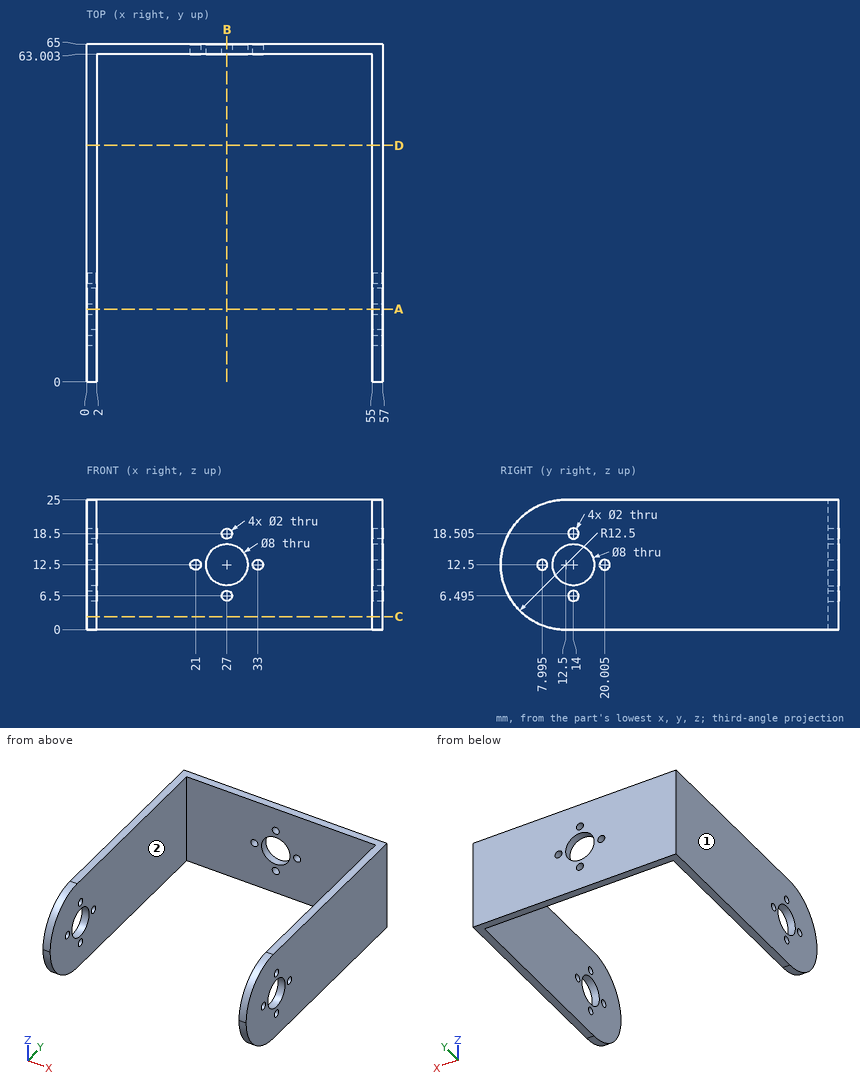
Could you check a few things on this drawing? It's one solid part, dimensions in mm from its lowest x, y, z. A direction names the side the tool comes from. Give positions to 0.01 mm unless a question says otherwise; leave off trailing zeros. Order: outer loops, then holes, each group sorted by start corner. A loop starts at its lowest first (then second) coordinate and runs counter-clockwise, first axis right, second up. Notation, with made-up numbers: (72, 37.25) -> (102, 37.25) arc R23 ccw to (102, 72.25) -> close; hole circle Ø5 at (50, -37). An arc over 180 degrees is marked (long way). Answer in a Markdown table with one row per item. Add a question column.
Item 1: Imagine slicing it at C-C (z = 2.5). List the corners of the cut face in (x, y) for me.
Item 2: I'm going to push a flat-ended pin straight in: P1, Ø3, axis at x = 27, z = 6.5, coming from the -Y side. Where does the tip first touch, or does it pass through?
Item 3: For the marked faces 1 and 2, which set-ups out of +Z, -Z, +X, -X, +Y, -Y let a thin tool reach every point of the face, with its end or its side?
Item 4: Imagine slicing it at B-B (x = 27). List the corners of the cut face in (y, z) for me.
Item 5: Please list where these lines run through material, in increasing order: probe 1 along X at (y, z) = (60.5, 12); probe 2 along Y at (x, z) = (49, 17.5).
Item 6: Imagine slicing it at D-D (y = 45.5). List the corners of the cut face in (x, z) for me, and give its area (3 significant figures).
Item 7: Imagine slicing it at A-A (y = 14). Count the separate pieces of the cut face and the enclosed holes in it.
Result:
| question | item | result |
|---|---|---|
| 1 | outline | (0, 5) -> (2, 5) -> (2, 63) -> (55, 63) -> (55, 5) -> (57, 5) -> (57, 65) -> (0, 65) -> close |
| 2 | P1 | y = 63 |
| 3 | face 1 | +Z, -Z, -X, +Y, -Y |
| 3 | face 2 | +Z, -Z, -Y |
| 4 | outline | (63, 0) -> (65, 0) -> (65, 5.5) -> (63, 5.5) -> close; (63, 7.5) -> (65, 7.5) -> (65, 8.5) -> (63, 8.5) -> close; (63, 16.5) -> (65, 16.5) -> (65, 17.5) -> (63, 17.5) -> close; (63, 19.5) -> (65, 19.5) -> (65, 25) -> (63, 25) -> close |
| 5 | probe 1 | 0 to 2, 55 to 57 |
| 5 | probe 2 | 63 to 65 |
| 6 | outline | (0, 0) -> (2, 0) -> (2, 25) -> (0, 25) -> close; (55, 0) -> (57, 0) -> (57, 25) -> (55, 25) -> close |
| 6 | area | 100 mm2 |
| 7 | separate pieces | 8 |
| 7 | enclosed holes | 0 |
